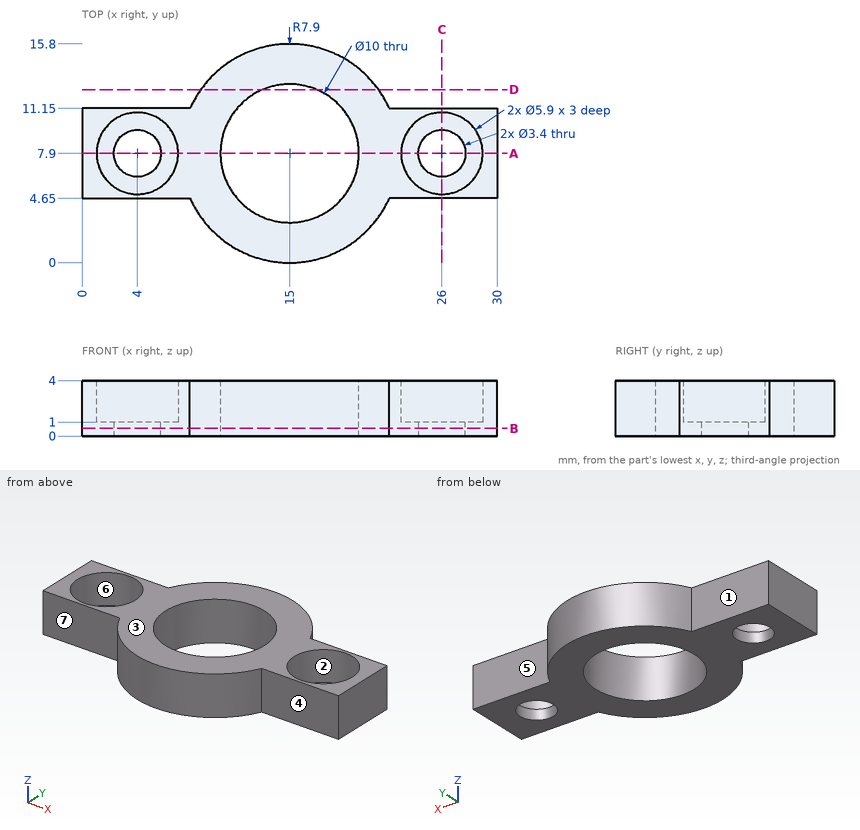
Drawing for the job (mm, zero at the part's lowest x, y, z). A direction names the side the tool comes from. Give positions to 0.01 mm unless a question says otherwise; leave off trailing zeros. Loops run counter-clockwise (first coordinate to the right, second up) from the corner with the lowest first, then second, coordinate; pieces in that order, holes last.
(1) Band-saw the part on A-A (y = 7.9). Write the cut outline in (x, z), and give its area (3 significant figures).
Return value:
outline: (0, 0) - (2.3, 0) - (2.3, 1) - (1.05, 1) - (1.05, 4) - (0, 4) - close; (5.7, 0) - (10, 0) - (10, 4) - (6.95, 4) - (6.95, 1) - (5.7, 1) - close; (20, 0) - (24.3, 0) - (24.3, 1) - (23.05, 1) - (23.05, 4) - (20, 4) - close; (27.7, 0) - (30, 0) - (30, 4) - (28.95, 4) - (28.95, 1) - (27.7, 1) - close
area: 37.8 mm2
(2) Band-saw the part on D-D (y = 12.5). Write the cut outline in (x, z), and give its area (3 significant figures).
Return value:
outline: (8.58, 0) - (13.04, 0) - (13.04, 4) - (8.58, 4) - close; (16.96, 0) - (21.42, 0) - (21.42, 4) - (16.96, 4) - close
area: 35.7 mm2
(3) Pin check, flat tips, straight feed: pin 1 (1.5 mm diameter, centred on y = 13, z = 1, fed in from +X); pin 2 (4 mm diameter, centred on x = 4, y = 7.9, fed in from +Z); pin 3 (2 mm diameter, centred on x = 25.5, y = 2, fed in from -Z); pin 4 (1 mm diameter, centred on x = 16, z = 1, fed in from -Y). Stop position of each tip, or through.
Return value:
pin 1: stops at x = 21.59
pin 2: stops at z = 1
pin 3: passes through
pin 4: stops at y = 0.02
(4) Drill centre lines: line 1 along Y through (x, z) = (15, 1); line 2 along X through (y, z) = (9.25, 2.6); line 3 along Y through (x, z) = (4, 0.3). Where is each one in solid material? Low to high.
Return value:
line 1: y = 0 to 2.9, 12.9 to 15.8
line 2: x = 0 to 1.38, 6.62 to 10.19, 19.81 to 23.38, 28.62 to 30
line 3: y = 4.65 to 6.2, 9.6 to 11.15
(5) Pull direction Y, two halves, no side cores. Call the marked faces 1, 2 and 3: pulls with the +Y half, pulls with the -Y half, needs draft (parallel to the pull), parting line crosses it, or undercut.
Return value:
face 1: pulls with the +Y half
face 2: undercut
face 3: needs draft
(6) Band-saw the part on C-C (x = 26). Write the cut outline in (y, z).
Return value:
outline: (4.65, 0) - (6.2, 0) - (6.2, 1) - (4.95, 1) - (4.95, 4) - (4.65, 4) - close; (9.6, 0) - (11.15, 0) - (11.15, 4) - (10.85, 4) - (10.85, 1) - (9.6, 1) - close
(7) 3-axis set-ups, long thin cutter, end or side, ignore diameter. For the marked faces 4, 5, 6 and 7: which of +Z, -Z, +X, -X, +Y, -Y reach the whole face in a straight line?
Return value:
face 4: +Z, -Z, +X, -Y
face 5: +Z, -Z, +X, +Y
face 6: +Z
face 7: +Z, -Z, -X, -Y
(8) Band-saw the part on B-B (z = 0.55). Write the cut outline in (x, y), and give its area (3 significant figures).
Return value:
outline: (0, 4.65) - (7.8, 4.65) arc R7.9 ccw to (22.2, 4.65) - (30, 4.65) - (30, 11.15) - (22.2, 11.15) arc R7.9 ccw to (7.8, 11.15) - (0, 11.15) - close; hole circle Ø3.4 at (4, 7.9); hole circle Ø10 at (15, 7.9); hole circle Ø3.4 at (26, 7.9)
area: 195 mm2
